Can you work these out from the model? Positions are in its coordinate system, mm. A direction names the side the tool comes from. Give positions to 0.01 mm unless a question says otherwise; leave off trailing zeros. Order: outer loops, then holes, each group sorted by start corner. A loop starts at its lowest first (then second) coordinate and runs counter-clockwise, first axis right, second up. Notation, with made-up numbers: (69.25, 3) - (76.25, 3) arc R19 ccw to (76.25, 32) - close; hole circle Ø10 at (2, 87). An arc over 180 degrees is marked (long way). Use one line per item in the form item = value. Start each with the question number.
1) For pin 1 (1.5 mm diameter, centred on x = -2.5, z = -5.5, fed in from -Y); pin 2 (1 mm diameter, centred on x = 4, z = -4, fed in from -Y), each with a flat end and sliding along its axis, tell me the tip position at first contact or that it passes through.
2) Please list where these lines run through material, in increasing order: probe 1 along Y at (x, z) = (0, -4.2); probe 2 along Y at (x, z) = (8.25, -3.15); probe 3 along Z at (x, y) = (6.25, 10).
3) Which directions (+Z, -Z, +X, -X, +Y, -Y) give clear straight access to the entire face, cutting with the end or side of a thin tool? Please do faces 1 (the flat face through (7.303, 1.653, -4.518)), 2 (the cylindrical face through (-7.335, 1.722, -5.929)), 3 (the cylindrical face through (-7.333, 1.718, -3.075)).
4) We'd pull the mould along X, two halves only. Please class faces 4 (the flat face through (0, 6, -6)), 5 (the cylindrical face through (7.422, 1.677, -3.075)), 6 (the cylindrical face through (0, 12, -5)): released by +X, released by -X, zero draft, split by the parting line, or undercut.
5) Suppose I cut it at B-B, the plane z = -4.5. Write out the boundary of the cut face in (x, y).
6) Suppose I cut it at A-A, the plane x = 0. Write out the boundary of the cut face in (y, z).
```python
from build123d import *

# Parameters (mm, degrees)
BOSS_EXTRUDE2_DEPTH = 3
FILLET2_R           = 1
FILLET3_R           = 0.25
SKETCH4_R           = 1
CUT_EXTRUDE1_DEPTH  = 10


with BuildPart() as part:
    # Sketch3 → Boss-Extrude2 (new body)
    with BuildSketch(Plane.XY.offset(-6)):
        with BuildLine():
            Line((4.165977905, 3.090909091), (11.989810158, -0.494421262))
            ThreePointArc((11.989810158, -0.494421262), (0, 12), (-11.989810158, -0.494421262))
            Line((-11.989810158, -0.494421262), (-4.165977905, 3.090909091))
            ThreePointArc((-4.165977905, 3.090909091), (0, 4), (4.165977905, 3.090909091))
        make_face()
    extrude(amount=BOSS_EXTRUDE2_DEPTH)

    # Fillet2
    fillet2_edges = [part.edges().sort_by_distance(p)[0] for p in [
        (11.989810158, -0.494421262, -4.5),
        (-11.989810158, -0.494421262, -4.5),
    ]]
    fillet(fillet2_edges, radius=FILLET2_R)

    # Fillet3
    fillet3_edges = [part.edges().sort_by_distance(p)[0] for p in [
        (0, 4, -3),
        (7.347934502, 1.632753394, -3),
        (-7.347934502, 1.632753394, -6),
        (-7.347934502, 1.632753394, -3),
        (0, 12, -6),
        (11.527432024, 0.26974446, -6),
        (-11.527432024, 0.26974446, -6),
        (0, 12, -3),
        (11.527432024, 0.26974446, -3),
        (-11.527432024, 0.26974446, -3),
        (7.347934502, 1.632753394, -6),
        (0, 4, -6),
    ]]
    fillet(fillet3_edges, radius=FILLET3_R)

    # Sketch4 → Cut-Extrude1 (cut)
    with BuildSketch(Plane(origin=(0, 0, -6), x_dir=(-1, 0, 0), z_dir=(0, 0, -1))):
        with Locations((0, 9.5)):
            Circle(SKETCH4_R)
        with Locations((8.6, 4)):
            Circle(SKETCH4_R)
        with Locations((-8.6, 4)):
            Circle(SKETCH4_R)
    extrude(amount=-CUT_EXTRUDE1_DEPTH, mode=Mode.SUBTRACT)


solid = part.part
```
Result sheet:
q1.pin_1 = 3.46
q1.pin_2 = 2.94
q2.probe_1 = 4 to 8.5, 10.5 to 12
q2.probe_2 = 1.24 to 3.06, 4.94 to 8.69
q2.probe_3 = -6 to -3
q3.face_1 = +Z, -Z, -Y
q3.face_2 = -Z, -Y
q3.face_3 = +Z, -Y
q4.face_4 = zero draft
q4.face_5 = undercut
q4.face_6 = split by the parting line
q5.outline = (-11.94, 1.18) arc R1 ccw to (-10.53, 0.17) - (-4.17, 3.09) arc R10 cw to (4.17, 3.09) - (10.53, 0.17) arc R1 ccw to (11.94, 1.18) arc R12 ccw to start; hole circle Ø2 at (-8.6, 4); hole circle Ø2 at (0, 9.5); hole circle Ø2 at (8.6, 4)
q6.outline = (4, -5.75) arc R0.25 ccw to (4.25, -6) - (8.5, -6) - (8.5, -3) - (4.25, -3) arc R0.25 ccw to (4, -3.25) - close; (10.5, -6) - (11.75, -6) arc R0.25 ccw to (12, -5.75) - (12, -3.25) arc R0.25 ccw to (11.75, -3) - (10.5, -3) - close
